Work out the finished part from the listing and answer in its coordinate system (mm). A direction names the side the tool comes from. Coordinates: 2 decimals unless noted, no trailing zeros. Write each loop counter-clockwise with the first axis right and the second up, starting at its lowest first coordinate (ties: lowest second). Pieces come first, ordered by that corner, then holes. Notation, with made-up numbers: (76.25, -8.5) - (99.25, -8.5) arc R24 cw to (99.25, 3.5) - close; hole circle Ø11 at (-25.5, -30). An arc over 180 degrees is marked (long way). One line per item, written item: value.
```python
from build123d import *

# Parameters (mm, degrees)
F0_R     = 27
F0_R_2   = 11
F1_DEPTH = 7


with BuildPart() as f1:
    # F0 (on Front) → F1 (new body)
    with BuildSketch(Plane.XZ):
        Circle(F0_R)
        with BuildLine():
            ThreePointArc((3, 24.819347), (17.67767, 17.67767), (24.819347, 3))
            ThreePointArc((24.819347, 3), (24.954796, 1.502717), (25, 0))
            ThreePointArc((25, 0), (24.954796, -1.502717), (24.819347, -3))
            ThreePointArc((24.819347, -3), (17.67767, -17.67767), (3, -24.819347))
            ThreePointArc((3, -24.819347), (0, -25), (-3, -24.819347))
            ThreePointArc((-3, -24.819347), (-17.67767, -17.67767), (-24.819347, -3))
            ThreePointArc((-24.819347, -3), (-25, 0), (-24.819347, 3))
            ThreePointArc((-24.819347, 3), (-17.67767, 17.67767), (-3, 24.819347))
            ThreePointArc((-3, 24.819347), (0, 25), (3, 24.819347))
        make_face(mode=Mode.SUBTRACT)
        with BuildLine():
            ThreePointArc((-12.649111, -3), (-13, 0), (-12.649111, 3))
            Line((-12.649111, 3), (-24.819347, 3))
            ThreePointArc((-24.819347, 3), (-25, 0), (-24.819347, -3))
            Line((-24.819347, -3), (-12.649111, -3))
        make_face()
        with BuildLine():
            ThreePointArc((-3, 12.649111), (0, 13), (3, 12.649111))
            Line((3, 12.649111), (3, 24.819347))
            ThreePointArc((3, 24.819347), (0, 25), (-3, 24.819347))
            Line((-3, 24.819347), (-3, 12.649111))
        make_face()
        with BuildLine():
            ThreePointArc((12.649111, 3), (12.91198, 1.510225), (13, 0))
            ThreePointArc((13, 0), (12.91198, -1.510225), (12.649111, -3))
            Line((12.649111, -3), (24.819347, -3))
            ThreePointArc((24.819347, -3), (24.954796, -1.502717), (25, 0))
            ThreePointArc((25, 0), (24.954796, 1.502717), (24.819347, 3))
            Line((24.819347, 3), (12.649111, 3))
        make_face()
        with BuildLine():
            ThreePointArc((12.649111, -3), (12.91198, -1.510225), (13, 0))
            ThreePointArc((13, 0), (12.91198, 1.510225), (12.649111, 3))
            ThreePointArc((12.649111, 3), (9.192388, 9.192388), (3, 12.649111))
            ThreePointArc((3, 12.649111), (0, 13), (-3, 12.649111))
            ThreePointArc((-3, 12.649111), (-9.192388, 9.192388), (-12.649111, 3))
            ThreePointArc((-12.649111, 3), (-13, 0), (-12.649111, -3))
            ThreePointArc((-12.649111, -3), (-9.192388, -9.192388), (-3, -12.649111))
            ThreePointArc((-3, -12.649111), (0, -13), (3, -12.649111))
            ThreePointArc((3, -12.649111), (9.192388, -9.192388), (12.649111, -3))
        make_face()
        Circle(F0_R_2, mode=Mode.SUBTRACT)
        with BuildLine():
            Line((3, -24.819347), (3, -12.649111))
            ThreePointArc((3, -12.649111), (0, -13), (-3, -12.649111))
            Line((-3, -12.649111), (-3, -24.819347))
            ThreePointArc((-3, -24.819347), (0, -25), (3, -24.819347))
        make_face()
    extrude(amount=F1_DEPTH)


solid = f1.part
```
Item 1: Which of the six approach directions +Z, -Z, +X, -X, +Y, -Y give full straight-line access (tool end or side, diameter ignored) to faces 1 (the face through (8, -7, -8)), 2 (the face through (17.842, -3.451, -17.512))?
Evaluation:
face 1: +Z, -Z, +X, -X, -Y
face 2: +Y, -Y
Item 2: Determine the mould class of faces 3 (the face through (-5.85, -3.45, -26.36)), 4 (the face through (8, 0, -8)), 5 (the face through (-9.121, -3.451, 9.263)), 6 (the face through (-3, -3, 19)) for opening direction X: +X half, -X half, draft (parallel to the pull), parting line (faces both ways), or undercut.
Evaluation:
face 3: parting line
face 4: draft
face 5: undercut
face 6: undercut
Item 3: Consider probe 1 along Z at (x, y) = (0, -5.5); probe 2 along Z at (x, y) = (3.5, -1.5); probe 3 along X at (y, z) = (-6, 13.5). Determine where each line is inside the solid, lowest interval first.
Evaluation:
probe 1: z = -27 to -11, 11 to 27
probe 2: z = -26.77 to -24.75, -12.52 to -10.43, 10.43 to 12.52, 24.75 to 26.77
probe 3: x = -23.38 to -21.04, -3 to 3, 21.04 to 23.38
Item 4: Given pin 1 (3.5 mm diameter, centred on x = 18.5, y = -2, fed in from +Z); pin 2 (4 mm diameter, centred on y = -4.5, z = -4, fed in from +X); pin 3 (2 mm diameter, centred on x = -18.5, y = -3.5, fed in from -Z), each flat-ended and moving along its own axis, determine where each tip first touches the part or whether it passes through.
Evaluation:
pin 1: stops at z = 21.18
pin 2: stops at x = 26.93
pin 3: stops at z = -20.56
Item 5: Section A-A, the plane z = 0 is taken. Determine the outline of the cut face in (x, y), then the cut area to 3 significant figures.
Evaluation:
outline: (-27, -7) - (-11, -7) - (-11, 0) - (-27, 0) - close; (11, -7) - (27, -7) - (27, 0) - (11, 0) - close
area: 224 mm2
Item 6: Section D-D, the plane x = -6.5 is taken. Determine the outline of the cut face in (y, z), then the cut area to 3 significant figures.
Evaluation:
outline: (-7, -26.21) - (0, -26.21) - (0, -24.14) - (-7, -24.14) - close; (-7, -11.26) - (0, -11.26) - (0, -8.87) - (-7, -8.87) - close; (-7, 8.87) - (0, 8.87) - (0, 11.26) - (-7, 11.26) - close; (-7, 24.14) - (0, 24.14) - (0, 26.21) - (-7, 26.21) - close
area: 62.3 mm2
Item 7: Section C-C, the plane y = -2 is taken. Determine the outline of the cut face in (x, z), then the cut area to 3 significant figures.
Evaluation:
outline: circle Ø54 at (0, 0); hole (-24.82, -3) arc R25 ccw to (-3, -24.82) - (-3, -12.65) arc R13 cw to (-12.65, -3) - close; hole (-24.82, 3) - (-12.65, 3) arc R13 cw to (-3, 12.65) - (-3, 24.82) arc R25 ccw to start; hole circle Ø22 at (0, 0); hole (3, -24.82) arc R25 ccw to (24.82, -3) - (12.65, -3) arc R13 cw to (3, -12.65) - close; hole (3, 12.65) arc R13 cw to (12.65, 3) - (24.82, 3) arc R25 ccw to (3, 24.82) - close
area: 767 mm2
Item 8: Section B-B, the plane x = 0 is taken. Determine the outline of the cut face in (y, z).
Evaluation:
outline: (-7, -27) - (0, -27) - (0, -11) - (-7, -11) - close; (-7, 11) - (0, 11) - (0, 27) - (-7, 27) - close
